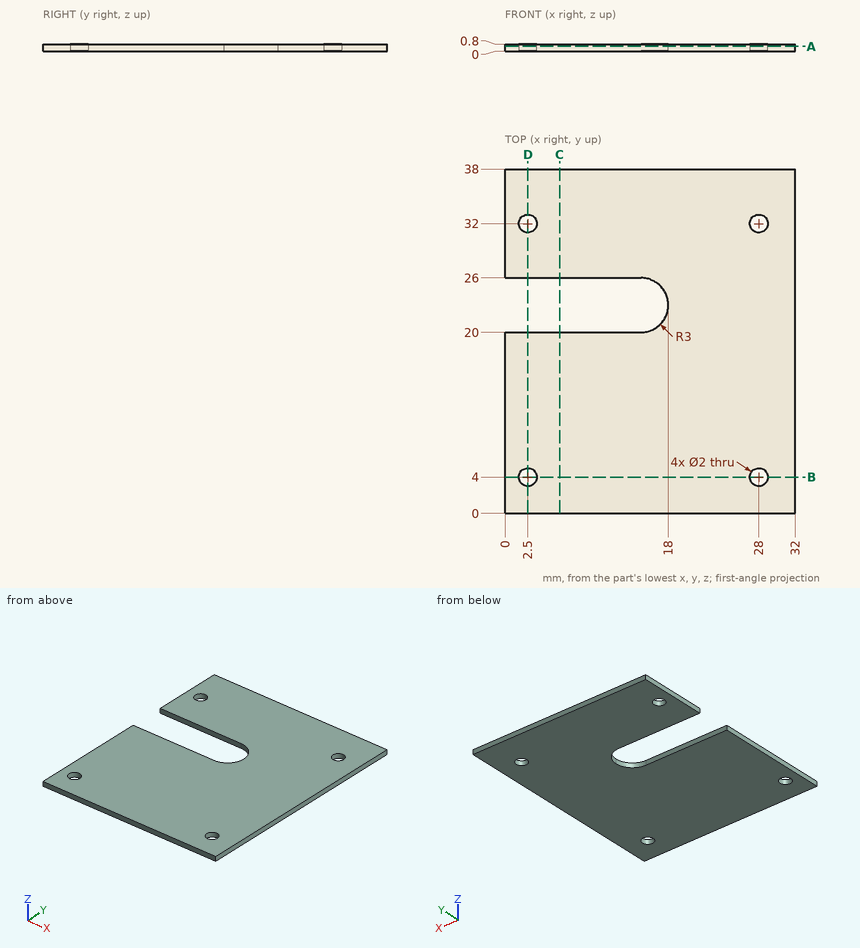
The drawing under review shows one solid part. Ordinate dimensions are in mm from its lowest x, y, z. Give positions to 0.01 mm unless a question says otherwise; leave off trailing zeros. Loops run counter-clockwise (first coordinate to the right, second up) from the corner with the lowest first, then second, coordinate; pieces in that order, holes last. Notation, with made-up numbers: M -10.5,58 L 33.5,58 A31 cw 33.5,86 Z; hole C 51.25,-7 d8. An arc over 180 degrees is marked long. One line per question, with ' | ' between items. Start each with the question number.
1. Insertion check: P1, Ø1.2, axis at x = 2.5, y = 4, coming from the -Z side. The pin has a flat end and moves straight along its axis. Give the tip position at first contact, or say it passes through.
2. Add section B-B (y = 4). Write out the cut boundary in (x, z).
3. Add section C-C (x = 6). Write out the cut boundary in (y, z), plus the area to 3 significant figures.
4. To check wall thickness, follow L1, parallel to Y at x = 28, z = 0.5; L2, parallel to Y at x = 2.5, z = 0.55; L3, parallel to X at y = 32, z = 0.2. State the ranges of each line that lie inside material, in increasing order.
5. Add section D-D (x = 2.5). Write out the cut boundary in (y, z).
6. Add section A-A (z = 0.55). Give the number of separate pieces and of enclosed holes in the cut face, plus the area to 3 significant figures.
Worked out:
1) P1: passes through
2) outline: M 0,0 L 1.5,0 L 1.5,0.8 L 0,0.8 Z; M 3.5,0 L 27,0 L 27,0.8 L 3.5,0.8 Z; M 29,0 L 32,0 L 32,0.8 L 29,0.8 Z
3) outline: M 0,0 L 20,0 L 20,0.8 L 0,0.8 Z; M 26,0 L 38,0 L 38,0.8 L 26,0.8 Z | area: 25.6 mm²
4) L1: y = 0 to 3, 5 to 31, 33 to 38 | L2: y = 0 to 3, 5 to 20, 26 to 31, 33 to 38 | L3: x = 0 to 1.5, 3.5 to 27, 29 to 32
5) outline: M 0,0 L 3,0 L 3,0.8 L 0,0.8 Z; M 5,0 L 20,0 L 20,0.8 L 5,0.8 Z; M 26,0 L 31,0 L 31,0.8 L 26,0.8 Z; M 33,0 L 38,0 L 38,0.8 L 33,0.8 Z
6) separate pieces: 1 | enclosed holes: 4 | area: 1,100 mm²
